```python
from build123d import *

# Parameters (mm, degrees)
BOX026_W          = 30
BOX026_H          = 20
BOX026_DEPTH      = 9.2
CYLINDER008_R     = 0.75
CYLINDER008_DEPTH = 7
ARRAY008_X_COUNT  = 10
ARRAY008_X_PITCH  = 2.6
ARRAY008_Y_COUNT  = 2
ARRAY008_Y_PITCH  = 1
BOX025_W          = 26
BOX025_H          = 12
BOX025_DEPTH      = 5.2
BOX024_W          = 26
BOX024_H          = 18
BOX024_DEPTH      = 7.2


with BuildPart() as obj1:
    # Box026 → Box026 (new body)
    with BuildSketch(Plane(origin=(-1, -1, 3.6), x_dir=(1, 0, 0), z_dir=(0, 0, 1))):
        with Locations((15, 10)):
            Rectangle(BOX026_W, BOX026_H)
    extrude(amount=BOX026_DEPTH)


with BuildPart() as array008:
    # Cylinder008 → Cylinder008 (new body)
    with BuildSketch(Plane(origin=(1.3, -1, 3.6), x_dir=(1, 0, 0), z_dir=(0, 1, 0))):
        Circle(CYLINDER008_R)
    extrude(amount=CYLINDER008_DEPTH)

    # Array008 X: Array008 ×10


with BuildPart() as array008_1:
    add(array008.part)
    with Locations(*[(i * ARRAY008_X_PITCH, 0, 0) for i in range(1, ARRAY008_X_COUNT)]):
        add(array008.part)

    # Array008 Y: Array008 ×2


with BuildPart() as array008_2:
    add(array008_1.part)
    with Locations(*[(0, i * ARRAY008_Y_PITCH, 0) for i in range(1, ARRAY008_Y_COUNT)]):
        add(array008_1.part)


with BuildPart() as cube_10_base011:
    # Box025 → Box025 (new body)
    with BuildSketch(Plane(origin=(0, 6, 1), x_dir=(1, 0, 0), z_dir=(0, 0, 1))):
        with Locations((13, 6)):
            Rectangle(BOX025_W, BOX025_H)
    extrude(amount=BOX025_DEPTH)


with BuildPart() as obj2:
    # Box024 → Box024 (new body)
    with BuildSketch(Plane.XY):
        with Locations((13, 9)):
            Rectangle(BOX024_W, BOX024_H)
    extrude(amount=BOX024_DEPTH)

    # Cut025: cut cube_10_base011
    add(cube_10_base011.part, mode=Mode.SUBTRACT)

    # Cut024: cut Array008
    add(array008_2.part, mode=Mode.SUBTRACT)

    # Cut027: cut obj1
    add(obj1.part, mode=Mode.SUBTRACT)


solid = obj2.part
```
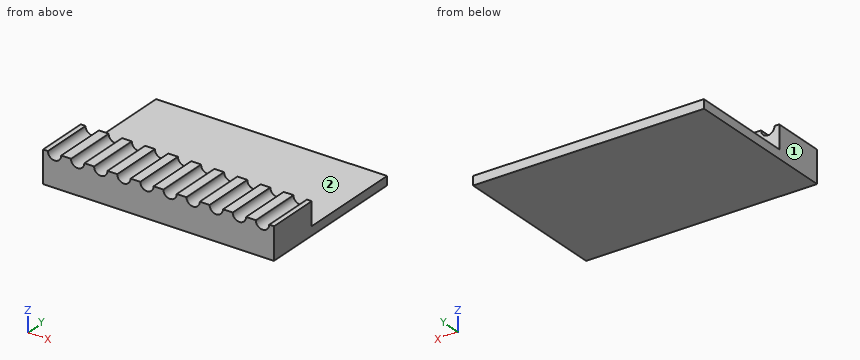
Verification items for the finished model (mm, model axes). Face numbers are marked on the shaded views. A direction names the side the tool comes from. Round coordinates to 2 decimals unless told otherwise and drop trailing zeros. Write each loop counter-clockwise with the first axis right and the second up, starting at its lowest first coordinate (ties: lowest second). Pieces come first, ordered by that corner, then holes. Notation, with made-up numbers: (52.25, -10.5) -> (68.25, -10.5) arc R14 ccw to (68.25, 3.5) -> close; hole circle Ø2 at (7, 71.5). An arc over 180 degrees is marked (long way). Write each question's results on one line, items separated by ' | '.
Q1. Thickness scan on probe 1 along Y at (x, z) = (12, 2.7); probe 2 along Z at (x, y) = (22, 9); probe 3 along Z at (x, y) = (20, 5.5). Record the ranges inside material, lowest first.
Derived:
probe 1: y = 0 to 6 | probe 2: z = 0 to 1 | probe 3: z = 0 to 3.04
Q2. Go/stop test with a flat-tipped pin: pin 1 Ø1.3 at (x, z) = (17, 2) entering from +Y. Record where the tip stops, or that it passes through.
Derived:
pin 1: stops at y = 6
Q3. Sectioned sample at B-B, the plane z = 2.55. Record the boundary of the cut face in (x, y).
Derived:
outline: (0, 0) -> (26, 0) -> (26, 6) -> (0, 6) -> close
Q4. Access from +Z, -Z, +X, -X, +Y, -Y to the whole of each face (thin tool, end or side, straight path). Record for the marked faces 1 and 2.
Derived:
face 1: +Z, -Z, -X, +Y, -Y | face 2: +Z, +X, -X, +Y
Q5. Sectioned sample at D-D, the plane x = 11.25. Record the boundary of the cut face in (y, z).
Derived:
outline: (0, 0) -> (18, 0) -> (18, 1) -> (6, 1) -> (6, 3) -> (0, 3) -> close
Q6. Sectioned sample at C-C, the plane y = 15.5. Record the boundary of the cut face in (x, z).
Derived:
outline: (0, 0) -> (26, 0) -> (26, 1) -> (0, 1) -> close
Q7. Sectioned sample at A-A, the plane x = 15.5. Record the boundary of the cut face in (y, z), and give its area (3 significant figures).
Derived:
outline: (0, 0) -> (18, 0) -> (18, 1) -> (6, 1) -> (6, 3.6) -> (0, 3.6) -> close | area: 33.6 mm²
